```python
from build123d import *

# Parameters (mm, degrees)
SKETCH1_W            = 198
SKETCH1_H            = 108
BOSS_EXTRUDE1_DEPTH  = 40
SKETCH4_W            = 181
SKETCH4_H            = 45
CUT_EXTRUDE2_DEPTH   = 10
CUT_EXTRUDE3_START   = -198
CUT_EXTRUDE3_DEPTH   = 198
BOSS_EXTRUDE11_DEPTH = 10
CUT_EXTRUDE12_DEPTH  = 198
CUT_EXTRUDE28_DEPTH  = 14.5
CUT_EXTRUDE29_DEPTH  = 14.5
CUT_EXTRUDE40_REACH  = 231.059
SKETCH12_R           = 3.15
CUT_EXTRUDE9_DEPTH   = 230.058944379
SKETCH13_R           = 4.5
CUT_EXTRUDE10_DEPTH  = 16.5
SKETCH14_R           = 4.5
CUT_EXTRUDE11_DEPTH  = 16.5
SKETCH41_R           = 2.9
CUT_EXTRUDE21_DEPTH  = 7
CUT_EXTRUDE22_DEPTH  = 10
CUT_EXTRUDE23_DEPTH  = 10
CUT_EXTRUDE35_DEPTH  = 55.4
CUT_EXTRUDE34_DEPTH  = 55.4
CUT_EXTRUDE36_DEPTH  = 55.4
SKETCH90_R           = 6.1
CUT_EXTRUDE38_DEPTH  = 17
SKETCH96_R           = 2
CUT_EXTRUDE39_DEPTH  = 230.058944379
SKETCH98_R           = 7.5
CUT_EXTRUDE41_DEPTH  = 4


with BuildPart() as part:
    # Sketch1 → Boss-Extrude1 (new body)
    with BuildSketch(Plane(origin=(0, 0, 0), x_dir=(1, 0, 0), z_dir=(0, 1, 0))):
        with Locations((99, 54)):
            Rectangle(SKETCH1_W, SKETCH1_H)
    extrude(amount=BOSS_EXTRUDE1_DEPTH)

    # Sketch4 → Cut-Extrude2 (cut)
    with BuildSketch(Plane(origin=(0, 0, 0), x_dir=(1, 0, 0), z_dir=(0, 1, 0))):
        with Locations((99, 54)):
            Rectangle(SKETCH4_W, SKETCH4_H)
    extrude(amount=CUT_EXTRUDE2_DEPTH, mode=Mode.SUBTRACT)

    # Sketch5 → Cut-Extrude3 (cut)
    with BuildSketch(Plane(origin=(198, 0, 0), x_dir=(0, 0, -1), z_dir=(1, 0, 0)).offset(CUT_EXTRUDE3_START)):
        Polygon((54, 40), (108, 34.657672686), (108, 40), align=None)
    extrude(amount=CUT_EXTRUDE3_DEPTH, mode=Mode.SUBTRACT)

    # Sketch53 → Boss-Extrude11 (add)
    with BuildSketch(Plane(origin=(0, 10, 0), x_dir=(-1, 0, 0), z_dir=(0, -1, 0))):
        Polygon((-8.5, 51.5), (-8.5, 31.5), (-39.5, 31.5), align=None)
        Polygon((-8.5, 56.5), (-8.5, 76.5), (-39.5, 76.5), align=None)
        Polygon((-158.5, 76.5), (-189.5, 56.5), (-189.5, 76.5), align=None)
        Polygon((-158.5, 31.5), (-189.5, 51.5), (-189.5, 31.5), align=None)
    extrude(amount=BOSS_EXTRUDE11_DEPTH)

    # Sketch18 → Cut-Extrude12 (cut)
    with BuildSketch(Plane(origin=(198, 0, 0), x_dir=(0, 0, -1), z_dir=(1, 0, 0))):
        Polygon((0, 34.657672686), (0, 40), (54, 40), align=None)
    extrude(amount=-CUT_EXTRUDE12_DEPTH, mode=Mode.SUBTRACT)

    # Izq → Cut-Extrude28 (cut)
    with BuildSketch(Plane(origin=(0, 28.012686094, -12.204810084), x_dir=(1, 0, 0), z_dir=(0, 0.9167660546215652, -0.39942458749256926))):
        Polygon((8.5, 48.862182113), (29.5, 70.132603179), (8.5, 70.132603179), align=None)
    cut_extrude28 = extrude(amount=-CUT_EXTRUDE28_DEPTH, mode=Mode.SUBTRACT)

    # Der → Cut-Extrude29 (cut)
    with BuildSketch(Plane(origin=(0, -11.144923858, -4.62106599), x_dir=(1, 0, 0), z_dir=(0, 0.9237421135716327, 0.38301502270043264))):
        Polygon((8.5, 51.290217599), (29.5, 29.097876578), (8.5, 29.097876578), align=None)
    cut_extrude29 = extrude(amount=-CUT_EXTRUDE29_DEPTH, mode=Mode.SUBTRACT)

    # Cut-Extrude40: up to this face of the body (flat: up to its plane)
    cut_extrude40_end = Plane(part.part.faces().sort_by_distance((99, 10, -54))[0])
    # Sketch97 → Cut-Extrude40 (cut, up to the picked face)
    with BuildSketch(Plane(origin=(0, 0, 0), x_dir=(1, 0, 0), z_dir=(0, 1, 0)), mode=Mode.PRIVATE) as cut_extrude40_sk1:
        Polygon((8.5, 57.5), (29.5, 76.5), (158.5, 76.5), (189.5, 56.5), (189.5, 51.5), (158.5, 31.5), (29.5, 31.5), (8.5, 51.5), align=None)
    cut_extrude40_tool1 = split(extrude(cut_extrude40_sk1.sketch, amount=CUT_EXTRUDE40_REACH, mode=Mode.PRIVATE), bisect_by=cut_extrude40_end, keep=Keep.BOTH, mode=Mode.PRIVATE)
    cut_extrude40 = cut_extrude40_tool1.solids().sort_by(Axis((96.82024, 0, -54.014019), (0, 1, 0)))[0]
    add(cut_extrude40, mode=Mode.SUBTRACT)

    # Mirror2: Cut-Extrude28, Cut-Extrude29, Cut-Extrude40 across plane
    add(cut_extrude28.mirror(Plane(origin=(99, 0, 0), x_dir=(0, 0, 1), z_dir=(1, 0, 0))), mode=Mode.SUBTRACT)
    add(cut_extrude29.mirror(Plane(origin=(99, 0, 0), x_dir=(0, 0, 1), z_dir=(1, 0, 0))), mode=Mode.SUBTRACT)
    add(cut_extrude40.mirror(Plane(origin=(99, 0, 0), x_dir=(0, 0, 1), z_dir=(1, 0, 0))), mode=Mode.SUBTRACT)

    # Sketch12 → Cut-Extrude9 (cut, through all)
    with BuildSketch(Plane(origin=(0, 40, 0), x_dir=(1, 0, 0), z_dir=(0, 1, 0))):
        with Locations(Location((19.7, 98.85, 0), (0, 0, 270))):
            Circle(SKETCH12_R)
        with Locations(Location((99.7, 9.15, 0), (0, 0, 270))):
            Circle(SKETCH12_R)
        with Locations(Location((179.7, 9.15, 0), (0, 0, 270))):
            Circle(SKETCH12_R)
        with Locations(Location((19.7, 9.15, 0), (0, 0, 270))):
            Circle(SKETCH12_R)
        with Locations(Location((99.7, 98.85, 0), (0, 0, 270))):
            Circle(SKETCH12_R)
        with Locations(Location((179.7, 98.85, 0), (0, 0, 270))):
            Circle(SKETCH12_R)
    extrude(amount=-CUT_EXTRUDE9_DEPTH, mode=Mode.SUBTRACT)

    # Sketch13 → Cut-Extrude10 (cut)
    with BuildSketch(Plane(origin=(0, 44.902839065, -4.442327104), x_dir=(1, 0, 0), z_dir=(0, 0.9951418638934392, -0.0984513622388844))):
        with Locations(Location((46.5, 91.063226213, 0), (0, 0, 270))):
            Circle(SKETCH13_R)
        with Locations(Location((151.5, 91.063226213, 0), (0, 0, 270))):
            Circle(SKETCH13_R)
    extrude(amount=-CUT_EXTRUDE10_DEPTH, mode=Mode.SUBTRACT)

    # Sketch14 → Cut-Extrude11 (cut)
    with BuildSketch(Plane(origin=(0, 34.032645471, 6.317746484), x_dir=(1, 0, 0), z_dir=(0, 0.995141863893439, 0.09845136223888487))):
        with Locations(Location((46.5, 19.393715592, 0), (0, 0, 270))):
            Circle(SKETCH14_R)
        with Locations(Location((151.5, 19.393715592, 0), (0, 0, 270))):
            Circle(SKETCH14_R)
    extrude(amount=-CUT_EXTRUDE11_DEPTH, mode=Mode.SUBTRACT)

    # Sketch41 → Cut-Extrude21 (cut)
    with BuildSketch(Plane(origin=(0, 0, 0), x_dir=(1, 0, 0), z_dir=(0, 1, 0))):
        with Locations(Location((139.5, 9, 0), (0, 0, 90))):
            Circle(SKETCH41_R)
        with Locations(Location((139.5, 99, 0), (0, 0, 90))):
            Circle(SKETCH41_R)
    extrude(amount=CUT_EXTRUDE21_DEPTH, mode=Mode.SUBTRACT)

    # Sketch42 → Cut-Extrude22 (cut)
    with BuildSketch(Plane.XY):
        with BuildLine():
            Line((142.3, 12.8), (152, 12.8))
            ThreePointArc((152, 12.8), (153.8, 11), (152, 9.2))
            Line((152, 9.2), (142.3, 9.2))
            ThreePointArc((142.3, 9.2), (140.5, 11), (142.3, 12.8))
        make_face()
    extrude(amount=-CUT_EXTRUDE22_DEPTH, mode=Mode.SUBTRACT)

    # Sketch43 → Cut-Extrude23 (cut)
    with BuildSketch(Plane(origin=(0, 0, -108), x_dir=(-1, 0, 0), z_dir=(0, 0, -1))):
        with BuildLine():
            Line((-55.7, 12.8), (-46, 12.8))
            ThreePointArc((-46, 12.8), (-44.2, 11), (-46, 9.2))
            Line((-46, 9.2), (-55.7, 9.2))
            ThreePointArc((-55.7, 9.2), (-57.5, 11), (-55.7, 12.8))
        make_face()
    extrude(amount=-CUT_EXTRUDE23_DEPTH, mode=Mode.SUBTRACT)

    # Sketch84 → Cut-Extrude35 (cut)
    with BuildSketch(Plane(origin=(0, 44.902839065, -4.442327104), x_dir=(1, 0, 0), z_dir=(0, 0.9951418638934392, -0.0984513622388844))):
        with BuildLine():
            Line((31.7, 53.899606161), (166.7, 53.899606161))
            ThreePointArc((166.7, 53.899606161), (168.467766953, 54.631839208), (169.2, 56.399606161))
            Line((169.2, 56.399606161), (169.2, 71.399606161))
            ThreePointArc((169.2, 71.399606161), (168.467766953, 73.167373114), (166.7, 73.899606161))
            Line((166.7, 73.899606161), (31.7, 73.899606161))
            ThreePointArc((31.7, 73.899606161), (29.932233047, 73.167373114), (29.2, 71.399606161))
            Line((29.2, 71.399606161), (29.2, 56.399606161))
            ThreePointArc((29.2, 56.399606161), (29.932233047, 54.631839208), (31.7, 53.899606161))
        make_face()
    extrude(amount=-CUT_EXTRUDE35_DEPTH, mode=Mode.SUBTRACT)

    # Sketch83 → Cut-Extrude34 (cut)
    with BuildSketch(Plane(origin=(0, 34.321747276, 3.395518666), x_dir=(1, 0, 0), z_dir=(0, 0.9951418638934391, 0.0984513622388849))):
        with BuildLine():
            Line((31.7, 53.57571514), (166.7, 53.57571514))
            ThreePointArc((166.7, 53.57571514), (168.467766953, 52.843482093), (169.2, 51.07571514))
            Line((169.2, 51.07571514), (169.2, 36.07571514))
            ThreePointArc((169.2, 36.07571514), (168.467766953, 34.307948187), (166.7, 33.57571514))
            Line((166.7, 33.57571514), (31.7, 33.57571514))
            ThreePointArc((31.7, 33.57571514), (29.932233047, 34.307948187), (29.2, 36.07571514))
            Line((29.2, 36.07571514), (29.2, 51.07571514))
            ThreePointArc((29.2, 51.07571514), (29.932233047, 52.843482093), (31.7, 53.57571514))
        make_face()
    extrude(amount=-CUT_EXTRUDE34_DEPTH, mode=Mode.SUBTRACT)

    # Sketch85 → Cut-Extrude36 (cut)
    with BuildSketch(Plane(origin=(0, 40, 0), x_dir=(1, 0, 0), z_dir=(0, 1, 0))):
        Polygon((0, 101.9), (6.1, 108), (0, 108), align=None)
        Polygon((0, 0), (6.1, 0), (0, 6.1), align=None)
        Polygon((198, 6.1), (191.9, 0), (198, 0), align=None)
        Polygon((198, 108), (191.9, 108), (198, 101.9), align=None)
    extrude(amount=-CUT_EXTRUDE36_DEPTH, mode=Mode.SUBTRACT)

    # Sketch90 → Cut-Extrude38 (cut)
    with BuildSketch(Plane(origin=(0, 40, 0), x_dir=(1, 0, 0), z_dir=(0, 1, 0))):
        with Locations(Location((19.7, 9.15, 0), (0, 0, 270))):
            Circle(SKETCH90_R)
        with Locations(Location((99.7, 9.15, 0), (0, 0, 270))):
            Circle(SKETCH90_R)
        with Locations(Location((179.7, 9.15, 0), (0, 0, 270))):
            Circle(SKETCH90_R)
        with Locations(Location((99.7, 98.85, 0), (0, 0, 270))):
            Circle(SKETCH90_R)
        with Locations(Location((179.7, 98.85, 0), (0, 0, 270))):
            Circle(SKETCH90_R)
        with Locations(Location((19.7, 98.85, 0), (0, 0, 270))):
            Circle(SKETCH90_R)
    extrude(amount=-CUT_EXTRUDE38_DEPTH, mode=Mode.SUBTRACT)

    # Sketch96 → Cut-Extrude39 (cut, through all)
    with BuildSketch(Plane(origin=(0, 0, 0), x_dir=(1, 0, 0), z_dir=(0, 1, 0))):
        with Locations(Location((15.45, 54, 0), (0, 0, 180))):
            Circle(SKETCH96_R)
        with Locations((185, 54)):
            Circle(SKETCH96_R)
    extrude(amount=CUT_EXTRUDE39_DEPTH, mode=Mode.SUBTRACT)

    # Sketch98 → Cut-Extrude41 (cut)
    with BuildSketch(Plane(origin=(0, 40, 0), x_dir=(1, 0, 0), z_dir=(0, 1, 0))):
        with Locations(Location((185, 54, 0), (0, 0, 270))):
            Circle(SKETCH98_R)
        with Locations(Location((15.45, 54, 0), (0, 0, 270))):
            Circle(SKETCH98_R)
    extrude(amount=-CUT_EXTRUDE41_DEPTH, mode=Mode.SUBTRACT)


solid = part.part
```
Geometry: final body of the model. Coordinates: model frame, mm. A direction names the side the tool comes from. Round coordinates to 2 decimals unless told otherwise and drop trailing zeros. Order: outer loops, then holes, each group sorted by start corner. A loop starts at its lowest first (then second) coordinate and runs counter-clockwise, first axis right, second up. Notation, with made-up numbers: (48.25, 43.25) - (95.25, 43.25) arc R13 ccw to (95.25, 67.25) - close; hole circle Ø7 at (-39.75, 19). An arc over 180 degrees is marked (long way). Write item = value, one per line. Start each with the question number.
Q1. Cut plane C-C on x = 99.7. Give the number of separate pieces and of enclosed holes in the cut face, and give its area (3 significant figures).
Q2. Pull-direction query (Y, two-part tool) for faces 6 (the flat face through (21.48, 6.04, -39.14)), 7 (the flat face through (151.56, 19.51, -93.5)), 8 (the cylindrical face through (29.913, 24.931, -57.385)); classes: +Y half, -Y half, draft (parallel to the pull), parting line (faces both ways), or undercut.
Q3. Access query for faces 1 (the cylindrical face through (183, 23, -54)), 2 (the flat face through (183.52, 2.362, -37.196)), 3 (the cylindrical face through (153.8, 11, -4.9)), 4 (the flat face through (194.9, 17.9, -105)), 5 (the cylindrical face through (168.487, 23.96, -32.125)). Directions: +Z, -Z, +X, -X, +Y, -Y. A direction counts if a zero-diameter tool reaches every point of the face in a straight line with its end or side. Return the directions, or none.
Q4. Ray query, line 1 (X direction, y = 38.9, z = -54); line 2 (X direction, y = 4, z = -9); line 3 (Z direction, x = 31, y = 7). Return the intervals inside material, ascending. Write a range as from..to.
Q5. Cut plane A-A on x = 79. Return the cut outline in (y, z).
Q6. Pin query (flat end, axial travel): pin 1 (7 mm diameter, centred on x = 179.7, z = -98.85, fed in from +Y); pin 2 (1.7 mm diameter, centred on x = 140, z = -97.5, fed in from -Y); pin 3 (6 mm diameter, centred on x = 20.5, z = -102, fed in from +Y). Return the tip coordinate at first contact, or that it passes through.
Q7. Cut plane B-B on z = -40.5. Return the cut outline in (x, y), and give its area (3 significant figures).
Outcome:
q1.separate_pieces = 5
q1.enclosed_holes = 0
q1.area = 1,840 mm^2
q2.face_6 = draft
q2.face_7 = undercut
q2.face_8 = -Y half
q3.face_1 = +Y, -Y
q3.face_2 = -Y
q3.face_3 = +Z
q3.face_4 = -Z, +X, +Y, -Y
q3.face_5 = +Y
q4.line_1 = 0..7.95, 22.95..177.5, 192.5..198
q4.line_2 = 0..16.55, 22.85..96.55, 102.85..136.6, 142.4..176.55, 182.85..198
q4.line_3 = -108..-76.5, -31.5..0
q5.outline = (0, -108) - (34.66, -108) - (37.63, -77.98) - (10, -75.25) - (10, -76.5) - (0, -76.5) - close; (0, -31.5) - (10, -31.5) - (10, -32.75) - (37.63, -30.02) - (34.66, 0) - (0, 0) - close; (10, -55.15) - (39.6, -58.08) - (40, -54) - (39.6, -49.92) - (10, -52.85) - close
q6.pin_1 = 23
q6.pin_2 = 7
q6.pin_3 = 35.02
q7.outline = (0, 0) - (8.5, 0) - (8.5, 3.73) - (20.05, 3.73) - (20.05, 10) - (29.2, 10) - (29.2, 38.66) - (0, 38.66) - close; (169.2, 10) - (177.95, 10) - (177.95, 3.73) - (189.5, 3.73) - (189.5, 0) - (198, 0) - (198, 38.66) - (169.2, 38.66) - close
q7.area = 1,980 mm^2
